CAD build for the part. Positions are in the model's coordinates, mm. Face numbers are marked on the shaded views. A direction names the side the tool comes from. Coordinates: 2 decimals unless noted, no trailing zeros. Order: outer loops, then holes, each group sorted by start corner. A loop starts at its lowest first (then second) coordinate and runs counter-clockwise, first axis right, second up.
from build123d import *

# Parameters (mm, degrees)
SKETCH1_W            = 1450
SKETCH1_H            = 880
BOSS_EXTRUDE1_DEPTH  = 40
SHELL1_T             = 3
SKETCH2_W            = 94
SKETCH2_H            = 30
CUT_EXTRUDE1_DEPTH   = 118
SKETCH3_W            = 37
SKETCH3_H            = 677
BOSS_EXTRUDE2_DEPTH  = 100
FILLET1_R            = 20
SKETCH4_R            = 19.494294984
CUT_EXTRUDE2_DEPTH   = 100
FILLET1_OF_MIRROR1_R = 20


with BuildPart() as part:
    # Sketch1 → Boss-Extrude1 (new, symmetric)
    with BuildSketch(Plane.XY):
        Rectangle(SKETCH1_W, SKETCH1_H)
    extrude(amount=BOSS_EXTRUDE1_DEPTH, both=True)

    # Shell1 (no face opened: a closed hollow body)
    add(offset(amount=-SHELL1_T, mode=Mode.PRIVATE), mode=Mode.SUBTRACT)

    # Sketch2 → Cut-Extrude1 (cut)
    with BuildSketch(Plane.XY):
        with Locations((-440, 295)):
            Rectangle(SKETCH2_W, SKETCH2_H)
        with Locations((440, 295)):
            Rectangle(SKETCH2_W, SKETCH2_H)
    extrude(amount=CUT_EXTRUDE1_DEPTH, mode=Mode.SUBTRACT)

    # Sketch3 → Boss-Extrude2 (add)
    with BuildSketch(Plane(origin=(725, 0, 0), x_dir=(0, 0, -1), z_dir=(1, 0, 0))):
        with Locations((18.5, 1.5)):
            Rectangle(SKETCH3_W, SKETCH3_H)
    boss_extrude2 = extrude(amount=BOSS_EXTRUDE2_DEPTH)

    # Fillet1
    fillet1_edges = [part.edges().sort_by_distance(p)[0] for p in [
        (775, 340, 0),
        (775, -337, 0),
        (825, 340, -18.5),
        (825, 1.5, 0),
        (825, -337, -18.5),
    ]]
    fillet(fillet1_edges, radius=FILLET1_R)

    # Sketch4 → Cut-Extrude2 (cut)
    with BuildSketch(Plane.XY):
        with Locations((765, 246.927736461)):
            Circle(SKETCH4_R)
        with Locations((765, 86.927736461)):
            Circle(SKETCH4_R)
        with Locations((765, -73.072263539)):
            Circle(SKETCH4_R)
        with Locations((765, -233.072263539)):
            Circle(SKETCH4_R)
    cut_extrude2 = extrude(amount=-CUT_EXTRUDE2_DEPTH, mode=Mode.SUBTRACT)

    # Mirror1: Boss-Extrude2, Cut-Extrude2 across plane
    add(boss_extrude2.mirror(Plane(origin=(0, 0, 0), x_dir=(0, 0, 1), z_dir=(1, 0, 0))))
    add(cut_extrude2.mirror(Plane(origin=(0, 0, 0), x_dir=(0, 0, 1), z_dir=(1, 0, 0))), mode=Mode.SUBTRACT)

    # Fillet1 of Mirror1
    fillet1_of_mirror1_edges = [part.edges().sort_by_distance(p)[0] for p in [
        (-775, 340, 0),
        (-775, -337, 0),
        (-825, 340, -18.5),
        (-825, 1.5, 0),
        (-825, -337, -18.5),
    ]]
    fillet(fillet1_of_mirror1_edges, radius=FILLET1_OF_MIRROR1_R)


solid = part.part
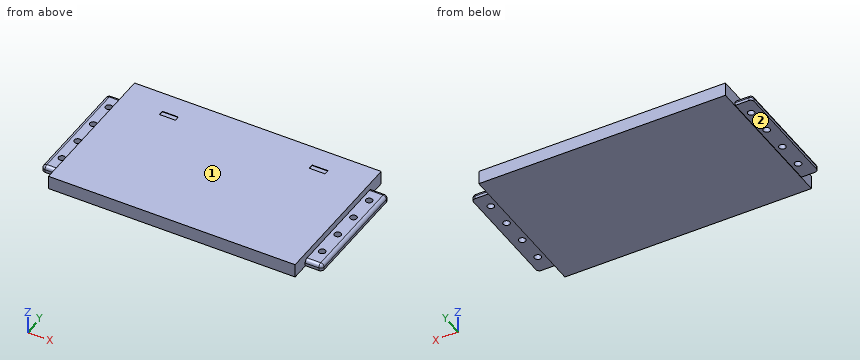
1) Slice it at A-A (y = 43). List the corners of the cut face in (x, z).
2) Pin check, flat tips, straight feed: P1, Ø8, axis at y = -44.5, z = -14, coming from the -X side; P2, Ø2, axis at y = 108, z = -4, coming from the -X side; P3, Ø13.5, axis at x = -762, z = -24.5, coming from the +Y side. Stop position of each tip, or through.
3) Slice it at B-B (x = 765). List the corners of the cut face in (y, z).
4) Which spindle directions (+Z, -Z, +X, -X, +Y, -Y) get a long thin tool onto all of the face, cutting with end or side? Do the marked faces 1 and 2. Say none if no direction does.
5) Drill centre lines: probe 1 along Y at (x, z) = (-765, -24.5); probe 2 along Y at (x, z) = (-569, 1.5); probe 3 along X at (y, z) = (-148.5, -31). Where is each one in solid material? Low to high.
Worked out:
1. outline: (-825, -37) - (-725, -37) - (-725, -40) - (725, -40) - (725, -37) - (825, -37) - (825, -20) arc R20 ccw to (805, 0) - (725, 0) - (725, 40) - (-725, 40) - (-725, 0) - (-805, 0) arc R20 ccw to (-825, -20) - close; hole (-722, -37) - (722, -37) - (722, 37) - (-722, 37) - close
2. P1: stops at x = -824.9
2. P2: stops at x = -818.23
2. P3: stops at y = 340
3. outline: (-337, -37) - (-252.57, -37) - (-252.57, 0) - (-317, 0) arc R20 ccw to (-337, -20) - close; (-213.58, -37) - (-92.57, -37) - (-92.57, 0) - (-213.58, 0) - close; (-53.58, -37) - (67.43, -37) - (67.43, 0) - (-53.58, 0) - close; (106.42, -37) - (227.43, -37) - (227.43, 0) - (106.42, 0) - close; (266.42, -37) - (340, -37) - (340, -20) arc R20 ccw to (320, 0) - (266.42, 0) - close
4. face 1: +Z, +X, -X, +Y, -Y
4. face 2: -Z, -X, +Y, -Y
5. probe 1: y = -337 to -252.57, -213.58 to -92.57, -53.58 to 67.43, 106.42 to 227.43, 266.42 to 340
5. probe 2: y = -440 to -437, 437 to 440
5. probe 3: x = -825 to -722, 722 to 825
